Read the model definition and answer for the solid it produces. Units are mm, in the model's axes. Face numbers are marked on the shaded views. Give positions to 0.01 mm unless a question says otherwise; leave off trailing zeros. Write each loop counter-clockwise with the first axis right and the second up, starting at its lowest first coordinate (ties: lowest second). Pieces come first, ordered by that corner, then holes. Notation, with made-up numbers: M 39,86.5 L 49,86.5 A18 cw 49,106.5 Z; hole C -22.75,71 d7. An arc over 180 degrees is marked long. Use a Markdown table: item, result. Add a question column.
Item 1: A cutting plane is placed at B-B on x = -21.5. Determine the outline of the cut face in (y, z).
Item 2: The mould has two halves that part along Z. Classify the marked faces 1, 2 and 3: pulls with the +Z half, pulls with the -Z half, needs draft (parallel to the pull), parting line crosses it, or undercut.
Item 3: Given P1, Ø8, axis at y = 30.5, z = 8.5, coming from the -X side; P2, Ø1.2, axis at y = 12.5, z = 6.5, coming from the +X side; P3, Ø8.5, axis at x = 0.5, z = -9.5, coming from the +Y side; P4, Ø25, axis at x = 16.5, y = 15, coming from the +Z side, each flat-ended and moving along its own axis, determine where each tip first touches the part or whether it passes through.
Item 4: A cutting plane is placed at A-A on x = 32.5. Determine the outline of the cut face in (y, z), then the cut area to 3 significant figures.
Item 5: Consider probe 1 along X at (y, z) = (-1.8, -16); probe 2 along X at (y, z) = (18, 1.5); probe 3 along Y at (x, z) = (-11, -17). Determine where each line is inside the solid, lowest interval first. Write a range as [from, to].
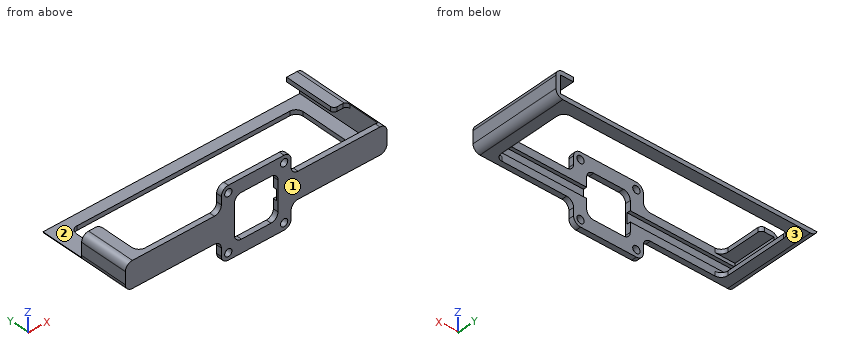
from build123d import *

# Parameters (mm, degrees)
BOSS_EXTRUDE1_DEPTH   = 50
BOSS_EXTRUDE1_2_DEPTH = 50
SKETCH2_W             = 130
SKETCH2_H             = 6.504238827
BOSS_EXTRUDE2_DEPTH   = 2.5
SKETCH4_R             = 2.1
SKETCH4_W             = 25
SKETCH4_H             = 25
BOSS_EXTRUDE4_DEPTH   = 3
FILLET1_R             = 4
SKETCH5_W             = 145
SKETCH5_H             = 6
CUT_EXTRUDE1_DEPTH    = 2
CUT_EXTRUDE2_DEPTH    = 5
SKETCH7_W             = 4.152825608
SKETCH7_H             = 25.088924328
CUT_EXTRUDE3_DEPTH    = 15
SKETCH8_W             = 11.5
SKETCH8_H             = 20
CUT_EXTRUDE5_DEPTH    = 5
FILLET2_R             = 2


with BuildPart() as part:
    # Sketch1 → Boss-Extrude1 (new body)
    with BuildSketch(Plane(origin=(0, 0, 0), x_dir=(1, 0, 0), z_dir=(0, 1, 0))):
        Polygon((-65, 5), (-65, 7.5), (-75, 7.5), (-75, -7.5), (-65, -7.5), (-65, -5), (-72.5, -5), (-72.5, 5), align=None)
    extrude(amount=BOSS_EXTRUDE1_DEPTH)



with BuildPart() as body_2:
    # Sketch1 → Boss-Extrude1 2 (new body)
    with BuildSketch(Plane(origin=(0, 0, 0), x_dir=(1, 0, 0), z_dir=(0, 1, 0))):
        Polygon((72.5, -5), (72.5, 5), (65, 5), (65, 7.5), (75, 7.5), (75, -7.5), (65, -7.5), (65, -5), align=None)
    extrude(amount=BOSS_EXTRUDE1_2_DEPTH)


with BuildPart() as part_1:
    add(part.part)

    add(body_2.part)  # Boss-Extrude2 merges body 2
    # Sketch2 → Boss-Extrude2 (add)
    with BuildSketch(Plane(origin=(0, 0, -7.5), x_dir=(-1, 0, 0), z_dir=(0, 0, -1))):
        with Locations((0, 46.747880587)):
            Rectangle(SKETCH2_W, SKETCH2_H)
    extrude(amount=-BOSS_EXTRUDE2_DEPTH)

    # Sketch4 → Boss-Extrude4 (add)
    with BuildSketch(Plane.XZ):
        Polygon((20, 7.5), (75, 7.5), (75, -7.5), (20, -7.5), (20, -20), (-20, -20), (-20, -7.5), (-75, -7.5), (-75, 7.5), (-20, 7.5), (-20, 20), (20, 20), align=None)
        with Locations(Location((16.001061443, 16.001061443, 0), (0, 0, 270))):
            Circle(SKETCH4_R, mode=Mode.SUBTRACT)
        with Locations(Location((-16, 16, 0), (0, 0, 270))):
            Circle(SKETCH4_R, mode=Mode.SUBTRACT)
        with Locations(Location((-16, -16, 0), (0, 0, 270))):
            Circle(SKETCH4_R, mode=Mode.SUBTRACT)
        with Locations(Location((16, -16, 0), (0, 0, 270))):
            Circle(SKETCH4_R, mode=Mode.SUBTRACT)
        with Locations((0.000530722, 0.000530722)):
            Rectangle(SKETCH4_W, SKETCH4_H, mode=Mode.SUBTRACT)
    extrude(amount=BOSS_EXTRUDE4_DEPTH)

    # Fillet1
    fillet1_edges = [part_1.edges().sort_by_distance(p)[0] for p in [
        (65, 0, 6.25),
        (75, 23.5, -7.5),
        (75, 23.5, 7.5),
        (65, 43.495761173, -6.25),
        (-65, 43.495761173, -6.25),
        (-65, 0, -6.25),
        (-75, 23.5, -7.5),
        (-75, 23.5, 7.5),
        (-65, 0, 6.25),
        (-20, -1.5, 7.5),
        (-20, -1.5, -7.5),
        (-20, -1.5, -20),
        (20, -1.5, -20),
        (20, -1.5, -7.5),
        (20, -1.5, 7.5),
        (20, -1.5, 20),
        (-20, -1.5, 20),
        (12.500530722, -1.5, 12.500530722),
        (-12.499469278, -1.5, 12.500530722),
        (-12.499469278, -1.5, -12.499469278),
        (12.500530722, -1.5, -12.499469278),
        (65, 0, -6.25),
    ]]
    fillet(fillet1_edges, radius=FILLET1_R)

    # Sketch5 → Cut-Extrude1 (cut)
    with BuildSketch(Plane(origin=(0, 0, 0), x_dir=(1, 0, 0), z_dir=(0, 1, 0))):
        Rectangle(SKETCH5_W, SKETCH5_H)
    extrude(amount=-CUT_EXTRUDE1_DEPTH, mode=Mode.SUBTRACT)

    # Sketch6 → Cut-Extrude2 (cut)
    with BuildSketch(Plane(origin=(-72.5, 0, 0), x_dir=(0, 0, -1), z_dir=(1, 0, 0))):
        Polygon((-14.532801633, 51.358122402), (-14.532801633, 25), (-5, 25), (5, 25), (5, 51.358122402), align=None)
    extrude(amount=-CUT_EXTRUDE2_DEPTH, mode=Mode.SUBTRACT)

    # Sketch7 → Cut-Extrude3 (cut)
    with BuildSketch(Plane.ZY.offset(72.5)):
        with Locations((7.076412804, 37.544462164)):
            Rectangle(SKETCH7_W, SKETCH7_H)
    extrude(amount=-CUT_EXTRUDE3_DEPTH, mode=Mode.SUBTRACT)

    # Sketch8 → Cut-Extrude5 (cut)
    with BuildSketch(Plane.XY.offset(7.5)):
        with Locations((66.75, 10)):
            Rectangle(SKETCH8_W, SKETCH8_H)
    extrude(amount=-CUT_EXTRUDE5_DEPTH, mode=Mode.SUBTRACT)

    # Fillet2
    fillet2_edges = [part_1.edges().sort_by_distance(p)[0] for p in [
        (72.5, 20, 6.104049622),
        (-65, 25, 6.25),
        (65, 20, 6.25),
    ]]
    fillet(fillet2_edges, radius=FILLET2_R)


solid = part_1.part
Filled in:
| question | item | result |
|---|---|---|
| 1 | outline | M -3,-8.38 L 0,-8.38 L 0,-3 L -2,-3 L -2,3 L 0,3 L 0,8.38 L -3,8.38 Z; M 43.5,-7.5 L 50,-7.5 L 50,-5 L 43.5,-5 Z |
| 2 | face 1 | needs draft |
| 2 | face 2 | undercut |
| 2 | face 3 | pulls with the -Z half |
| 3 | P1 | x = 65 |
| 3 | P2 | x = 74.2 |
| 3 | P3 | y = 50 |
| 3 | P4 | through |
| 4 | outline | M -3,-7.5 L 0,-7.5 L 0,-3 L -2,-3 L -2,3 L 0,3 L 0,7.5 L -3,7.5 Z; M 43.5,-7.5 L 50,-7.5 L 50,-5 L 43.5,-5 Z |
| 4 | area | 49.3 mm² |
| 5 | probe 1 | [-20, -18.1], [-13.9, 13.9], [18.1, 20] |
| 5 | probe 2 | [-75, -72.5], [72.5, 75] |
| 5 | probe 3 | [-3, 0] |
